```python
from build123d import *

# Parameters (mm, degrees)
SKETCH_1_W               = 25
SKETCH_1_H               = 35
SKETCH_1_R               = 8.5
EXTRUDE_4_DEPTH          = 2
HOLE_WIZARD_M3_1_D       = 2.5
PATTERN_CIRCULAR_1_COUNT = 2


with BuildPart() as part:
    # 스케치1 → 보스-돌출4 (new body)
    with BuildSketch(Plane(origin=(0, 0, 0), x_dir=(1, 0, 0), z_dir=(0, 1, 0))):
        Rectangle(SKETCH_1_W, SKETCH_1_H)
        Circle(SKETCH_1_R, mode=Mode.SUBTRACT)
    extrude(amount=EXTRUDE_4_DEPTH)

    # M3 탭을 위한 탭 드릴1 (through all)
    with Locations(Plane(origin=(0, 2, 0), x_dir=(1, 0, 0), z_dir=(0, 1, 0))):
        with Locations((0, 13)):
            hole_wizard_m3_1 = Hole(HOLE_WIZARD_M3_1_D / 2)

    # 원형 패턴1: M3 탭을 위한 탭 드릴1 ×2 about axis
    pattern_circular_1_axis = Axis((0, 0, 0), (0, 1, 0))
    for i in range(1, PATTERN_CIRCULAR_1_COUNT):
        add(hole_wizard_m3_1.rotate(pattern_circular_1_axis, i * 360 / PATTERN_CIRCULAR_1_COUNT), mode=Mode.SUBTRACT)


solid = part.part
```
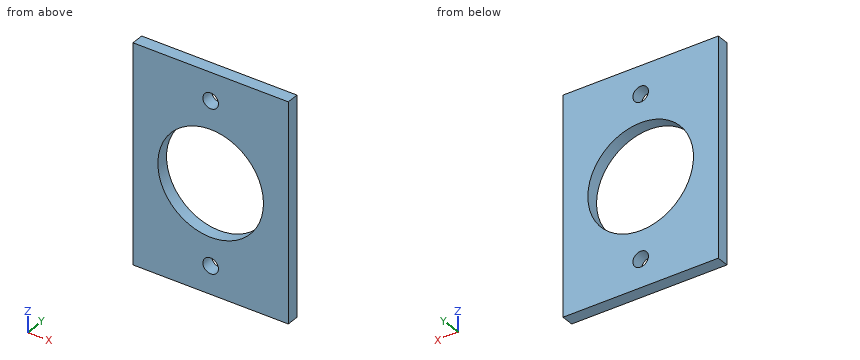
Geometry: final body of the model. Coordinates: model frame, mm. Round coordinates to 2 decimals unless told otherwise and drop trailing zeros. Write each loop counter-clockwise with the first axis right and the second up, starting at its lowest first coordinate (ties: lowest second). Pieces come first, ordered by that corner, then holes. Notation, with made-up numbers: (-37.75, 35) -> (4.25, 35) arc R30 cw to (4.25, 64) -> close; hole circle Ø5 at (59.25, 59.25). An arc over 180 degrees is marked (long way). Return JSON: item names as keys, results as strings.
Q1. Section A-A on z = 13. Return the cut outline in (x, y).
From the geometry:
{"outline": "(-12.5, 0) -> (-1.25, 0) -> (-1.25, 2) -> (-12.5, 2) -> close; (1.25, 0) -> (12.5, 0) -> (12.5, 2) -> (1.25, 2) -> close"}
Q2. Section B-B on x = 0. Return the cut outline in (y, z), and give its area (3 significant figures).
From the geometry:
{"outline": "(0, -17.5) -> (2, -17.5) -> (2, -14.25) -> (0, -14.25) -> close; (0, -11.75) -> (2, -11.75) -> (2, -8.5) -> (0, -8.5) -> close; (0, 8.5) -> (2, 8.5) -> (2, 11.75) -> (0, 11.75) -> close; (0, 14.25) -> (2, 14.25) -> (2, 17.5) -> (0, 17.5) -> close", "area": "26.0 mm2"}
Q3. First-contact query: pin 1 Ø10 at (x, z) = (0, 0) entering from -Y. Flat tip, straight axial feed; report the tip coordinate or a pass-through.
From the geometry:
{"pin 1": "through"}
Q4. Section D-D on z = 0. Return the cut outline in (x, y), and give its area (3 significant figures).
From the geometry:
{"outline": "(-12.5, 0) -> (-8.5, 0) -> (-8.5, 2) -> (-12.5, 2) -> close; (8.5, 0) -> (12.5, 0) -> (12.5, 2) -> (8.5, 2) -> close", "area": "16.0 mm2"}
Q5. Ray query, line 1 (Z direction, x = 0, y = 1.45); line 2 (X direction, y = 0.6, z = -13); line 3 (Z direction, x = 0.75, y = 1.85). Return the intervals inside material, ascending.
From the geometry:
{"line 1": "-17.5 to -14.25, -11.75 to -8.5, 8.5 to 11.75, 14.25 to 17.5", "line 2": "-12.5 to -1.25, 1.25 to 12.5", "line 3": "-17.5 to -14, -12 to -8.47, 8.47 to 12, 14 to 17.5"}
Q6. Section C-C on y = 1.4. Return the cut outline in (x, z), and give its area (3 significant figures).
From the geometry:
{"outline": "(-12.5, -17.5) -> (12.5, -17.5) -> (12.5, 17.5) -> (-12.5, 17.5) -> close; hole circle Ø17 at (0, 0); hole circle Ø2.5 at (0, -13); hole circle Ø2.5 at (0, 13)", "area": "638 mm2"}
